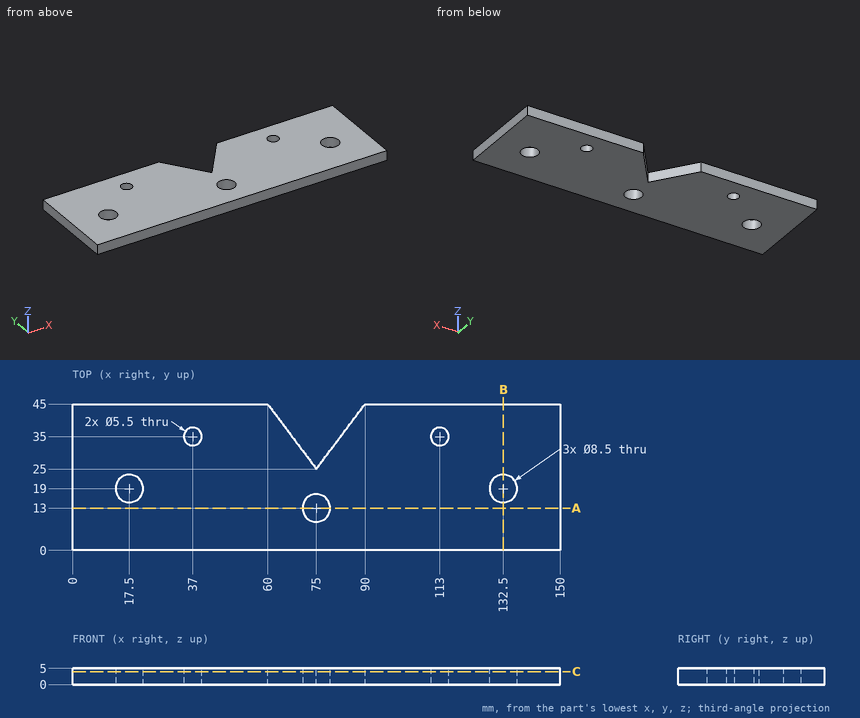
Study the drawing (mm; zero at the part's minimum x, y, z) and answer. Coordinates: 2 decimals unless noted, no trailing zeros. Write each loop counter-clockwise with the first axis right and the second up, starting at its lowest first coordinate (ties: lowest second). Pieces come first, ordered by that corner, then holes. Notation, with made-up numbers: (85.25, 80) - (117.25, 80) arc R27 ccw to (117.25, 115) - close; hole circle Ø7 at (30.25, 8). An arc over 180 degrees is marked (long way). Put each result on its own line as item: value.
1. Find the intervals of material crossed by line 1 along Y through (x, z) = (37, 1.9); line 2 along Y through (x, z) = (132.5, 2); line 3 along X through (y, z) = (20, 3.5), in increasing order. Write a range as from..to.
Answer sheet:
line 1: y = 0..32.25, 37.75..45
line 2: y = 0..14.75, 23.25..45
line 3: x = 0..13.37, 21.63..128.37, 136.63..150
2. The part is cut by section C-C on z = 4. Give the vertices of the cut face in (x, y).
Answer sheet:
outline: (0, 0) - (150, 0) - (150, 45) - (90, 45) - (75, 25) - (60, 45) - (0, 45) - close; hole circle Ø8.5 at (17.5, 19); hole circle Ø5.5 at (37, 35); hole circle Ø8.5 at (75, 13); hole circle Ø5.5 at (113, 35); hole circle Ø8.5 at (132.5, 19)
3. A flat-ended cylindrical pin translates along its axis: pin 1 Ø1 at (x, z) = (63, 1) entering from +Y. Find the tip coordinate at first contact, or state that the pin passes through.
Answer sheet:
pin 1: stops at y = 41.67
4. The part is cut by section A-A on y = 13. Give the vertices of the cut face in (x, z).
Answer sheet:
outline: (0, 0) - (70.75, 0) - (70.75, 5) - (0, 5) - close; (79.25, 0) - (150, 0) - (150, 5) - (79.25, 5) - close
5. The part is cut by section B-B on x = 132.5. Give the vertices of the cut face in (y, z).
Answer sheet:
outline: (0, 0) - (14.75, 0) - (14.75, 5) - (0, 5) - close; (23.25, 0) - (45, 0) - (45, 5) - (23.25, 5) - close
